The listing builds one solid part. Answer for the finished solid, in the listing's coordinates (mm). A direction names the side the tool comes from. Coordinates: 2 decimals unless noted, no trailing zeros. Write each loop counter-clockwise with the first axis right and the second up, starting at its lowest first coordinate (ties: lowest second). Pieces come first, ordered by that corner, then holes.
```python
from build123d import *

# Parameters (mm, degrees)
F2_R     = 12.5
F3_DEPTH = 253.15408
F4_SIZE  = 3.175
F5_R     = 3.175


with BuildPart() as f1:
    # F0 (on Top) → F1 (revolve)
    with BuildSketch(Plane.XY):
        Polygon((-118.936889, 48.041679), (-118.936889, 0), (110.082783, 0), (110.082783, 24.608025), (60.65549, 24.608025), (60.65549, 35.83255), (-30.912993, 35.83255), (-30.912993, 48.041679), align=None)
    revolve(axis=Axis((-4.427053, 0, 0), (1, 0, 0)))

    # F2 (on face) → F3 (cut)
    with BuildSketch(Plane(origin=(-118.936889, 0, 0), x_dir=(0, -1, 0), z_dir=(-1, 0, 0))):
        Circle(F2_R)
    extrude(amount=-F3_DEPTH, mode=Mode.SUBTRACT)

    # F4
    f4_edges = [f1.edges().sort_by_distance(p)[0] for p in [
        (-118.936889, -48.041679, 0),
        (-30.912993, -48.041679, 0),
        (60.65549, -35.83255, 0),
        (110.082783, -24.608025, 0),
    ]]
    chamfer(f4_edges, length=F4_SIZE)

    # F5
    f5_edges = [f1.edges().sort_by_distance(p)[0] for p in [
        (60.65549, -24.608025, 0),
        (-30.912993, -35.83255, 0),
    ]]
    fillet(f5_edges, radius=F5_R)


solid = f1.part
```
(1) Each of these flat-tipped pins is pushed along its axis until it touches: pin 1 (3 mm diameter, centred on x = 23.5, y = -31, fed in from -Z); pin 2 (8 mm diameter, centred on x = -82.5, z = -36.5, fed in from +Y); pin 3 (1 mm diameter, centred on x = -12, y = 23.5, fed in from -Z). Where does it stop, or does it pass through?
(2) Find the intervals of material crossed by probe 1 along Z at (x, y) = (37, 0); probe 2 along Z at (x, y) = (-54.5, 0); probe 3 along X at (y, z) = (37, 24.5), in increasing order.
(3) Section C-C, the plane x = 26 is taken. Write down the section's boundary in (y, z).
(4) Which of the six approach directions +Z, -Z, +X, -X, +Y, -Y give full straight-line access (tool end or side, diameter ignored) to faces 1 (the flat face through (-30.913, 14, 37)), 2 (the cylindrical face through (-75.5, -10.41, -46.9))?
(5) For a pull along Y with two mould halves and no side action, classify faces 3 (the flat face through (110.083, -9, -9)), 4 (the cylindrical face through (-6.03, -11.923, 3.755)), 5 (the conical face through (-118.74, 20.79, -39.98)) as pulls with the +Y half, pulls with the -Y half, needs draft (parallel to the pull), parting line crosses it, or undercut.
(6) Section D-D, the plane x = -38 is taken. Write down the section's boundary in (y, z), plus the area to 3 significant figures.
Solution:
1. pin 1: stops at z = -20.34
1. pin 2: stops at y = 35.38
1. pin 3: stops at z = -27.48
2. probe 1: z = -35.83 to -12.5, 12.5 to 35.83
2. probe 2: z = -48.04 to -12.5, 12.5 to 48.04
2. probe 3: x = -118.94 to -30.91
3. outline: circle Ø71.67 at (0, 0); hole circle Ø25 at (0, 0)
4. face 1: +X
4. face 2: +X, -X
5. face 3: needs draft
5. face 4: undercut
5. face 5: parting line crosses it
6. outline: circle Ø96.08 at (0, 0); hole circle Ø25 at (0, 0)
6. area: 6,760 mm2
